```python
from build123d import *

# Parameters (mm, degrees)
SKETCH1_W                                  = 700
SKETCH1_H                                  = 700
BOSS_EXTRUDE1_DEPTH                        = 10
SKETCH2_R                                  = 4
SKETCH2_W                                  = 115
SKETCH2_H                                  = 55
CUT_EXTRUDE2_DEPTH                         = 10
FILLET1_R                                  = 4
MIRROR3_AT_THE_SECOND_PLANE_COPY_1_SKETC_R = 4
MIRROR3_AT_THE_SECOND_PLANE_COPY_1_SKETC_W = 115
MIRROR3_AT_THE_SECOND_PLANE_COPY_1_SKETC_H = 55
MIRROR3_AT_THE_SECOND_PLANE_COPY_1_DEPTH   = 10
FILLET2_R                                  = 4
SKETCH3_R                                  = 2.1
SKETCH3_R_2                                = 1.6
CUT_EXTRUDE3_DEPTH                         = 991
SKETCH4_W                                  = 10
SKETCH4_H                                  = 20
SKETCH4_W_2                                = 15
CUT_EXTRUDE4_DEPTH                         = 991


with BuildPart() as part:
    # Sketch1 → Boss-Extrude1 (new body)
    with BuildSketch(Plane(origin=(0, 0, 0), x_dir=(1, 0, 0), z_dir=(0, 1, 0))):
        with Locations((350, 350)):
            Rectangle(SKETCH1_W, SKETCH1_H)
    extrude(amount=BOSS_EXTRUDE1_DEPTH)

    # Sketch2 → Cut-Extrude2 (cut)
    with BuildSketch(Plane(origin=(0, 10, 0), x_dir=(1, 0, 0), z_dir=(0, 1, 0))):
        with Locations(Location((88.9, 110, 0), (0, 0, 270))):
            Circle(SKETCH2_R)
        with Locations(Location((128.9, 110, 0), (0, 0, 270))):
            Circle(SKETCH2_R)
        with Locations(Location((128.9, 100, 0), (0, 0, 270))):
            Circle(SKETCH2_R)
        with Locations(Location((88.9, 100, 0), (0, 0, 270))):
            Circle(SKETCH2_R)
        with Locations((108.9, 47.5)):
            Rectangle(SKETCH2_W, SKETCH2_H)
    cut_extrude2 = extrude(amount=-CUT_EXTRUDE2_DEPTH, mode=Mode.SUBTRACT)

    # Fillet1
    fillet1_edges = [part.edges().sort_by_distance(p)[0] for p in [
        (51.4, 5, -75),
        (166.4, 5, -75),
        (166.4, 5, -20),
        (51.4, 5, -20),
    ]]
    fillet(fillet1_edges, radius=FILLET1_R)

    # Mirror3: Cut-Extrude2 across plane
    add(cut_extrude2.mirror(Plane.XY.offset(-350)), mode=Mode.SUBTRACT)

    # Mirror3 at the second plane: Cut-Extrude2 across plane
    add(cut_extrude2.mirror(Plane.ZY.offset(-350)), mode=Mode.SUBTRACT)

    # Mirror3 at the second plane copy 1 sketc → Mirror3 at the second plane copy 1 (cut)
    with BuildSketch(Plane(origin=(700, 10, -700), x_dir=(-1, 0, 0), z_dir=(0, 1, 0))):
        with Locations(Location((88.9, 110, 0), (0, 0, 270))):
            Circle(MIRROR3_AT_THE_SECOND_PLANE_COPY_1_SKETC_R)
        with Locations(Location((128.9, 110, 0), (0, 0, 270))):
            Circle(MIRROR3_AT_THE_SECOND_PLANE_COPY_1_SKETC_R)
        with Locations(Location((128.9, 100, 0), (0, 0, 270))):
            Circle(MIRROR3_AT_THE_SECOND_PLANE_COPY_1_SKETC_R)
        with Locations(Location((88.9, 100, 0), (0, 0, 270))):
            Circle(MIRROR3_AT_THE_SECOND_PLANE_COPY_1_SKETC_R)
        with Locations((108.9, 47.5)):
            Rectangle(MIRROR3_AT_THE_SECOND_PLANE_COPY_1_SKETC_W, MIRROR3_AT_THE_SECOND_PLANE_COPY_1_SKETC_H)
    extrude(amount=-MIRROR3_AT_THE_SECOND_PLANE_COPY_1_DEPTH, mode=Mode.SUBTRACT)

    # Fillet2
    fillet2_edges = [part.edges().sort_by_distance(p)[0] for p in [
        (166.4, 5, -625),
        (51.4, 5, -625),
        (51.4, 5, -680),
        (166.4, 5, -680),
        (648.6, 5, -625),
        (533.6, 5, -625),
        (533.6, 5, -680),
        (648.6, 5, -680),
        (533.6, 5, -75),
        (648.6, 5, -75),
        (648.6, 5, -20),
        (533.6, 5, -20),
    ]]
    fillet(fillet2_edges, radius=FILLET2_R)

    # Sketch3 → Cut-Extrude3 (cut, through all)
    with BuildSketch(Plane(origin=(0, 10, 0), x_dir=(1, 0, 0), z_dir=(0, 1, 0))):
        with Locations(Location((470.208152802, 639.913780286, 0), (0, 0, 270))):
            Circle(SKETCH3_R)
        with Locations(Location((60.086219714, 229.791847198, 0), (0, 0, 90))):
            Circle(SKETCH3_R)
        with Locations(Location((639.913780286, 470.208152802, 0), (0, 0, 90))):
            Circle(SKETCH3_R)
        with Locations(Location((429.195959493, 598.901586978, 0), (0, 0, 270))):
            Circle(SKETCH3_R)
        with Locations(Location((388.183766184, 557.889393669, 0), (0, 0, 270))):
            Circle(SKETCH3_R)
        with Locations(Location((347.171572875, 516.87720036, 0), (0, 0, 270))):
            Circle(SKETCH3_R)
        with Locations(Location((306.159379566, 475.865007051, 0), (0, 0, 270))):
            Circle(SKETCH3_R)
        with Locations(Location((265.147186258, 434.852813742, 0), (0, 0, 270))):
            Circle(SKETCH3_R)
        with Locations(Location((224.134992949, 393.840620434, 0), (0, 0, 270))):
            Circle(SKETCH3_R)
        with Locations(Location((183.12279964, 352.828427125, 0), (0, 0, 270))):
            Circle(SKETCH3_R)
        with Locations(Location((142.110606331, 311.816233816, 0), (0, 0, 270))):
            Circle(SKETCH3_R)
        with Locations(Location((101.098413022, 270.804040507, 0), (0, 0, 270))):
            Circle(SKETCH3_R)
        with Locations(Location((229.791847198, 60.086219714, 0), (0, 0, 270))):
            Circle(SKETCH3_R)
        with Locations(Location((270.804040507, 101.098413022, 0), (0, 0, 90))):
            Circle(SKETCH3_R)
        with Locations(Location((311.816233816, 142.110606331, 0), (0, 0, 90))):
            Circle(SKETCH3_R)
        with Locations(Location((352.828427125, 183.12279964, 0), (0, 0, 90))):
            Circle(SKETCH3_R)
        with Locations(Location((393.840620434, 224.134992949, 0), (0, 0, 90))):
            Circle(SKETCH3_R)
        with Locations(Location((434.852813742, 265.147186258, 0), (0, 0, 90))):
            Circle(SKETCH3_R_2)
        with Locations(Location((475.865007051, 306.159379566, 0), (0, 0, 90))):
            Circle(SKETCH3_R)
        with Locations(Location((516.87720036, 347.171572875, 0), (0, 0, 90))):
            Circle(SKETCH3_R)
        with Locations(Location((557.889393669, 388.183766184, 0), (0, 0, 90))):
            Circle(SKETCH3_R)
        with Locations(Location((598.901586978, 429.195959493, 0), (0, 0, 90))):
            Circle(SKETCH3_R)
    extrude(amount=-CUT_EXTRUDE3_DEPTH, mode=Mode.SUBTRACT)

    # Sketch4 → Cut-Extrude4 (cut, through all)
    with BuildSketch(Plane(origin=(0, 10, 0), x_dir=(1, 0, 0), z_dir=(0, 1, 0))):
        with Locations((602.5, 315)):
            Rectangle(SKETCH4_W, SKETCH4_H)
        with Locations((602.5, 185)):
            Rectangle(SKETCH4_W, SKETCH4_H)
        with Locations((567.5, 315)):
            Rectangle(SKETCH4_W, SKETCH4_H)
        with Locations((567.5, 185)):
            Rectangle(SKETCH4_W, SKETCH4_H)
        with Locations((537.5, 250)):
            Rectangle(SKETCH4_W_2, SKETCH4_H)
        with Locations((632.5, 250)):
            Rectangle(SKETCH4_W_2, SKETCH4_H)
    extrude(amount=-CUT_EXTRUDE4_DEPTH, mode=Mode.SUBTRACT)


solid = part.part
```
Model file for the job. Use its own axes, mm. Coordinates: 2 decimals unless noted, no trailing zeros. Answer as a JSON object with one key per item and string values. Group by question number.
1) Drill centre lines: L1, parallel to Z at x = 617, y = 3; L2, parallel to Z at x = 627.5, y = 9.5; L3, parallel to X at y = 0.5, z = -643. Where is each one in solid material? Low to high.
2) Flat gauge pin, fed straight in: pin 1 (2.5 mm diameter, centred on x = 516.88, z = -347.17, fed in from -Y). Where does the tip first touch, or does it go through?
3) Cut at A-A, the plane y = 7.25. Count the separate pieces of the cut face and the enclosed holes in it, then the cut area to 3 significant figures.
Check values:
{
 "1": {"L1": "z = -700 to -680, -625 to -75, -20 to 0", "L2": "z = -700 to -680, -625 to -260, -240 to -75, -20 to 0", "L3": "x = 0 to 51.4, 166.4 to 533.6, 648.6 to 700"},
 "2": {"pin 1": "passes through"},
 "3": {"separate pieces": "1", "enclosed holes": "48", "area": "462,000 mm²"}
}
